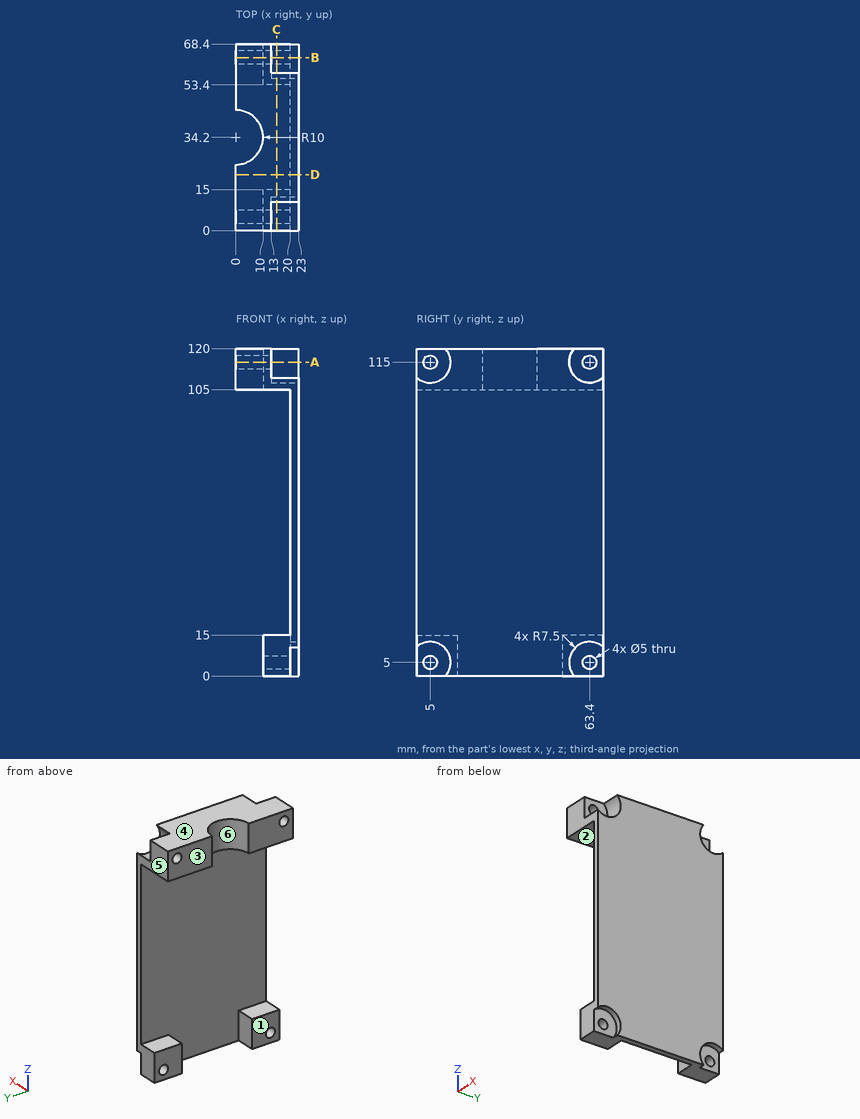
Answer from the drawing. Dimensions are ordinates in mm from the lowest x, y and z of the part. A direction names the side the tool comes from. Coordinates: 2 decimals unless noted, no trailing zeros. Loops run counter-clockwise (first coordinate to the right, second up) from the corner with the lowest first, then second, coordinate; pieces in that order, holes last. Notation, with made-up numbers: (58.5, -18.75) -> (98.5, -18.75) arc R27 cw to (98.5, 9.25) -> close; hole circle Ø6 at (75.25, 67.25). An arc over 180 degrees is marked (long way). Answer in a Markdown table with one row per item.
Item 1: Straight lines are drawn through the part: line 1 along Y through (x, z) = (12.5, 5); line 2 along Y through (x, z) = (8, 115); line 3 along X through (y, z) = (21.5, 82). For each, find the intervals that lie inside material, in ascending order. Write a range as [from, to].
Returned:
| item | result |
|---|---|
| line 1 | y = [0, 2.5], [7.5, 15], [53.4, 60.9], [65.9, 68.4] |
| line 2 | y = [0, 2.5], [7.5, 28.2], [40.2, 60.9], [65.9, 68.4] |
| line 3 | x = [20, 23] |
Item 2: A cutting plane is placed at D-D on y = 20.5. Determine the outline of the cut face in (x, z).
Returned:
| item | result |
|---|---|
| outline | (0, 105) -> (20, 105) -> (20, 0) -> (23, 0) -> (23, 120) -> (0, 120) -> close |
Item 3: A cutting plane is placed at A-A on z = 115. Determine the outline of the cut face in (x, y), plus the area to 3 significant figures.
Returned:
| item | result |
|---|---|
| outline | (0, 0) -> (13, 0) -> (13, 2.5) -> (0, 2.5) -> close; (0, 7.5) -> (13, 7.5) -> (13, 12.5) -> (23, 12.5) -> (23, 55.9) -> (13, 55.9) -> (13, 60.9) -> (0, 60.9) -> (0, 44.2) arc R10 cw to (0, 24.2) -> close; (0, 65.9) -> (13, 65.9) -> (13, 68.4) -> (0, 68.4) -> close |
| area | 1,040 mm^2 |
Item 4: For the marked faces 1, 2 and 3, determine the directions among +Z, -Z, +X, -X, +Y, -Y from which every point of the face is accessible in a straight line to the end or side of a thin tool.
Returned:
| item | result |
|---|---|
| face 1 | -Z, -X, +Y, -Y |
| face 2 | -X, +Y, -Y |
| face 3 | +Z, -Z, -X, +Y, -Y |
Item 5: Each of these flat-tipped pins is pushed along its axis until it touches: P1, Ø6, axis at y = 6, z = 5.5, coming from the +X side; P2, Ø16.5, axis at y = 59, z = 5.5, coming from the -X side; P3, Ø4, axis at y = 5, z = 115, coming from the +X side; P4, Ø6, axis at y = 63.5, z = 111, coming from the +X side. Where does it stop, or does it pass through?
Returned:
| item | result |
|---|---|
| P1 | stops at x = 20 |
| P2 | stops at x = 10 |
| P3 | passes through |
| P4 | stops at x = 13 |
Item 6: For a pull along Y with two mould halves and no side action, classify the marked faces 4, 5 and 6 as released by +Y, released by -Y, zero draft, split by the parting line, or undercut.
Returned:
| item | result |
|---|---|
| face 4 | zero draft |
| face 5 | released by +Y |
| face 6 | undercut |
Item 7: A cutting plane is placed at C-C on x = 15. Determine the outline of the cut face in (y, z), plus the area to 3 significant figures.
Returned:
| item | result |
|---|---|
| outline | (0, 0) -> (15, 0) -> (15, 15) -> (0, 15) -> close; (0, 105) -> (68.4, 105) -> (68.4, 109.41) arc R7.5 cw to (57.81, 120) -> (10.59, 120) arc R7.5 cw to (0, 109.41) -> close; (53.4, 0) -> (68.4, 0) -> (68.4, 15) -> (53.4, 15) -> close; hole circle Ø5 at (5, 5); hole circle Ø5 at (63.4, 5) |
| area | 1,160 mm^2 |
Item 8: A cutting plane is placed at B-B on y = 63.4. Determine the outline of the cut face in (x, z).
Returned:
| item | result |
|---|---|
| outline | (0, 105) -> (20, 105) -> (20, 15) -> (10, 15) -> (10, 7.5) -> (20, 7.5) -> (20, 12.5) -> (23, 12.5) -> (23, 107.5) -> (13, 107.5) -> (13, 112.5) -> (0, 112.5) -> close; (0, 117.5) -> (13, 117.5) -> (13, 120) -> (0, 120) -> close; (10, 0) -> (20, 0) -> (20, 2.5) -> (10, 2.5) -> close |
